Geometry: final body of the model. Coordinates: model frame, mm. Face numbers are marked on the shaded views. A direction names the side the tool comes from. Give positions to 0.01 mm unless a question says otherwise; leave off trailing zeros. Write each loop counter-clockwise with the first axis right and the second up, starting at its lowest first coordinate (ties: lowest second). Pieces come first, ordered by that corner, then holes. Notation, with made-up numbers: (18, 23.25) -> (28, 23.25) arc R14 ccw to (28, 40.25) -> close; hole circle Ø2 at (-3, -16). An arc over 180 degrees is marked (long way). Answer in a Markdown table with one row per item. Add a question column.
Item 1: Material intervals for probe 1 along Z at (x, y) = (36, -26); probe 2 along X at (y, z) = (-25.8, -15); probe 3 along Y at (x, z) = (3.1, 15), sorted ascending. Write a range as from..to.
Item 2: Section query A-A on z = -15. Output: boundary loops of the cut face in (x, y), plus the area to 3 significant figures.
Item 3: Section query B-B on y = 8. Output: boundary loops of the cut face in (x, z), plus the area to 3 significant figures.
Item 4: Section query D-D on x = 5. Output: boundary loops of the cut face in (y, z).
Item 5: First-contact query: P1, Ø8, axis at y = -11.5, z = -13.5, coming from the +X side; P2, Ø7.5, axis at y = 8, z = -15, coming from the -X side; P3, Ø1, axis at x = 50, z = -3.5, coming from the +Y side. Flat tips, straight axial feed; report the tip coordinate or a pass-through.
Item 6: Section query C-C on x = 36. Output: boundary loops of the cut face in (y, z), plus the area to 3 significant figures.
Item 7: Access query for the marked faces 1 and 2. Directions: +Z, -Z, +X, -X, +Y, -Y. A direction counts if a zero-diameter tool reaches every point of the face in a straight line with its end or side. Return the directions, or none.
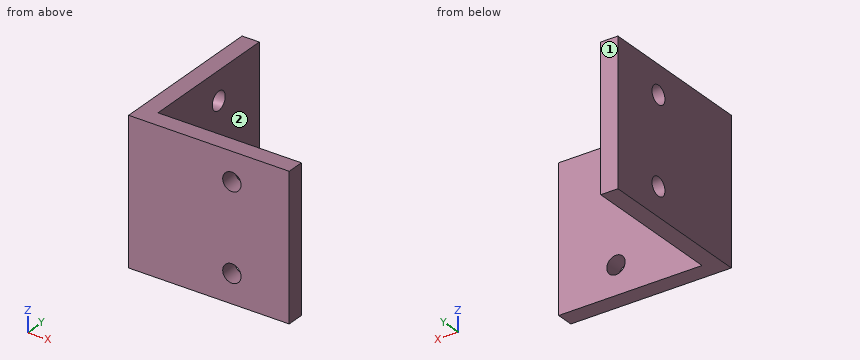
Autodesk Inventor part; units mm, degrees
ref_plane "YZ Plane" through (0, 0, 0) normal (1, 0, 0) x (0, 1, 0)
ref_plane "XZ Plane" through (0, 0, 0) normal (0, 1, 0) x (-1, 0, 0)
ref_plane "XY Plane" through (0, 0, 0) normal (0, 0, 1) x (1, 0, 0)
sketch "Sketch1" plane through (0, 0, 0) normal (1, 0, 0) x (0, 1, 0)
  line L0 (-28, 25) -> (28, 25)
  line L1 (28, 25) -> (28, -25)
  line L2 (28, -25) -> (-28, -25)
  line L3 (-28, -25) -> (-28, 25)
  line L4 (-28, 25) -> (28, -25) construction
  line L5 (28, 25) -> (-28, -25) construction
  point P0 (0, 0)
  dimension "d0" = 56
  dimension "d1" = 50
extrude "Extrusion1" add sketch "Sketch1" along normal blind 6
sketch "Sketch2" plane through (6, 0, 0) normal (1, 0, 0) x (0, 0, -1)
  line L0 (-25, -28) -> (25, -28)
  line L1 (25, -28) -> (25, -22)
  line L2 (25, -22) -> (-25, -22)
  line L3 (-25, -22) -> (-25, -28)
  point P0 (0, 0)
  dimension "d4" = 50
  dimension "d5" = 6
extrude "Extrusion2" add sketch "Sketch2" along normal blind 50
sketch "Sketch3" plane through (56, -22, 25) normal (0, 1, 0) x (1, 0, 0)
  circle A0 centre (-20, 10) radius 3.2
  circle A1 centre (-20, 40) radius 3.2
  point P0 (-56, 25)
  dimension "d9" = 6.4
  dimension "d10" = 6.4
sketch "Sketch4" plane through (6, 0, 0) normal (1, 0, 0) x (0, 0, -1)
  circle A0 centre (-15, 8) radius 3.2
  circle A1 centre (15, 8) radius 3.2
  point P0 (0, 0)
  dimension "d11" = 6.4
  dimension "d12" = 6.4
extrude "Extrusion3" cut sketch "Sketch4" against normal through all
extrude "Extrusion4" cut sketch "Sketch3" against normal through all
properties part number "Angle"
Findings below:
| question | item | result |
|---|---|---|
| 1 | probe 1 | z = -25..-18.2, -11.8..11.8, 18.2..25 |
| 1 | probe 2 | x = 0..32.8, 39.2..56 |
| 1 | probe 3 | y = -28..4.8, 11.2..28 |
| 2 | outline | (0, -28) -> (32.8, -28) -> (32.8, -22) -> (6, -22) -> (6, 4.8) -> (0, 4.8) -> close; (0, 11.2) -> (6, 11.2) -> (6, 28) -> (0, 28) -> close; (39.2, -28) -> (56, -28) -> (56, -22) -> (39.2, -22) -> close |
| 2 | area | 559 mm^2 |
| 3 | outline | (0, -25) -> (6, -25) -> (6, -18.2) -> (0, -18.2) -> close; (0, -11.8) -> (6, -11.8) -> (6, 11.8) -> (0, 11.8) -> close; (0, 18.2) -> (6, 18.2) -> (6, 25) -> (0, 25) -> close |
| 3 | area | 223 mm^2 |
| 4 | outline | (-28, -25) -> (28, -25) -> (28, 25) -> (-28, 25) -> close; hole circle Ø6.4 at (8, -15); hole circle Ø6.4 at (8, 15) |
| 5 | P1 | stops at x = 6 |
| 5 | P2 | stops at x = 0 |
| 5 | P3 | stops at y = -22 |
| 6 | outline | (-28, -25) -> (-22, -25) -> (-22, -18.2) -> (-28, -18.2) -> close; (-28, -11.8) -> (-22, -11.8) -> (-22, 11.8) -> (-28, 11.8) -> close; (-28, 18.2) -> (-22, 18.2) -> (-22, 25) -> (-28, 25) -> close |
| 6 | area | 223 mm^2 |
| 7 | face 1 | +Z, -Z, +X, -X, +Y |
| 7 | face 2 | +Z, -Z, +X, +Y |
